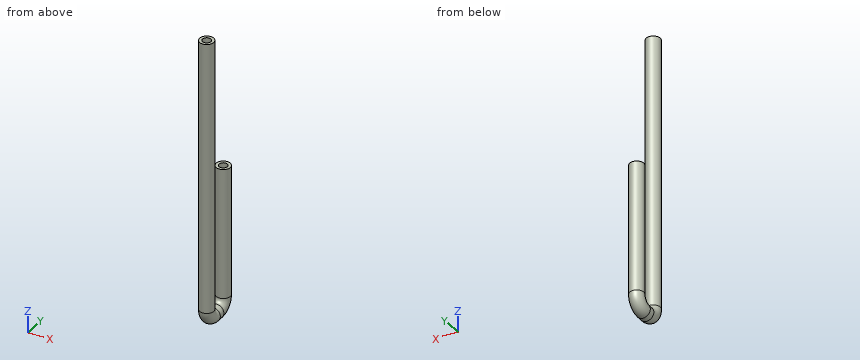
from build123d import *

# Parameters (mm, degrees)
SKETCH13_R   = 6.35
SKETCH13_R_2 = 3.81


with BuildPart() as part:
    # Sweep1: sweep along a path in Sketch14
    with BuildLine(Plane(origin=(0, 0, 0), x_dir=(0, 0, -1), z_dir=(1, 0, 0))) as sweep1_path:
        Line((0, -5.183219143), (117, -5.183219143))
        ThreePointArc((117, -5.183219143), (124.071067812, -8.112151331), (127, -15.183219143))
        Line((127, -15.183219143), (127, -20.583219143))
        ThreePointArc((127, -20.583219143), (124.071067812, -27.654286955), (117, -30.583219143))
        Line((117, -30.583219143), (-127, -30.583219143))
    # Sketch13 → Sweep1 (sweep)
    with BuildSketch(Plane.XY):
        with Locations((-0.83021259, -5.183219143)):
            Circle(SKETCH13_R)
        with Locations((-0.83021259, -5.183219143)):
            Circle(SKETCH13_R_2, mode=Mode.SUBTRACT)
    sweep(path=sweep1_path.line)


solid = part.part
Source: CAD feature listing. Evaluate the final solid. Frame: model axes, mm. Coordinates: 2 decimals unless noted, no trailing zeros. Write each loop counter-clockwise with the first axis right and the second up, starting at its lowest first coordinate (ties: lowest second). Pieces come first, ordered by that corner, then holes. Notation, with made-up numbers: M 17,35 L 67,35 A13 cw 67,46 Z; hole C -18,82.25 d3. An arc over 180 degrees is marked long. Use a Markdown table: item, result.
1) First-contact query: pin 1 Ø5 at (y, z) = (-8.5, -90) entering from +X; pin 2 Ø6 at (x, z) = (-3.5, -99) entering from -Y; pin 3 Ø3 at (x, y) = (-3.5, -13.5) entering from -Z; pin 4 Ø1.5 at (x, y) = (-5.5, -7.5) entering from -Z. Flat tips, straight axial feed; report the tip coordinate or a pass-through.
Conclusion:
| item | result |
|---|---|
| pin 1 | stops at x = 5.47 |
| pin 2 | stops at y = -36.93 |
| pin 3 | stops at z = -133.18 |
| pin 4 | stops at z = -130 |
2) Section A-A, the plane x = 1. Output: boundary loops of the cut face in (y, z), then the cut area to 3 significant figures.
Conclusion:
| item | result |
|---|---|
| outline | M -36.66,-117 A16.08 ccw -20.58,-133.08 L -15.18,-133.08 A16.08 ccw 0.9,-117 L 0.9,0 L -1.84,0 L -1.84,-117 A13.34 cw -15.18,-130.34 L -20.58,-130.34 A13.34 cw -33.92,-117 L -33.92,127 L -36.66,127 Z; M -27.24,-117 A6.66 ccw -20.58,-123.66 L -15.18,-123.66 A6.66 ccw -8.52,-117 L -8.52,0 L -11.26,0 L -11.26,-117 A3.92 cw -15.18,-120.92 L -20.58,-120.92 A3.92 cw -24.5,-117 L -24.5,127 L -27.24,127 Z |
| area | 2,180 mm^2 |
3) Section B-B, the plane z = -96. Output: boundary loops of the cut face in (x, y).
Conclusion:
| item | result |
|---|---|
| outline | C -0.83,-30.58 d12.7; C -0.83,-5.18 d12.7; hole C -0.83,-30.58 d7.62; hole C -0.83,-5.18 d7.62 |
4) Ray query, L1, parallel to Y at x = -4, z = -115.5; L2, parallel to Y at x = -1.25, z = -93.5; L3, parallel to Z at x = -1.5, y = -21. Return the intervals inside material, ascending.
Conclusion:
| item | result |
|---|---|
| L1 | y = -36.09 to -32.7, -28.47 to -25.08, -10.69 to -7.3, -3.07 to 0.32 |
| L2 | y = -36.92 to -34.37, -26.8 to -24.25, -11.52 to -8.97, -1.4 to 1.15 |
| L3 | z = -133.31 to -130.74, -123.24 to -120.66 |
5) Section C-C, the plane z = 45. Output: boundary loops of the cut face in (x, y), then the cut area to 3 significant figures.
Conclusion:
| item | result |
|---|---|
| outline | C -0.83,-30.58 d12.7; hole C -0.83,-30.58 d7.62 |
| area | 81.1 mm^2 |
